from build123d import *

# Parameters (mm, degrees)
F1_DEPTH = 4.826
F3_DEPTH = 2.921
F5_DEPTH = 2.921
F7_DEPTH = 25.4
F8_R     = 3.302
F9_R     = 6.35


with BuildPart() as f1:
    # F0 (on Top) → F1 (new body)
    with BuildSketch(Plane.XY):
        Polygon((-9.795272, 20.32), (-15.24, 0), (15.24, 0), (9.795272, 20.32), align=None)
    extrude(amount=F1_DEPTH)

    # F2 (on face) → F3 (join)
    with BuildSketch(Plane.XY.offset(4.826)):
        Polygon((-19.841803, 0), (19.841803, 0), (12.185154, 28.575), (-12.185154, 28.575), align=None)
    extrude(amount=F3_DEPTH)

    # F4 (on face) → F5 (join)
    with BuildSketch(Plane(origin=(0, 0, 0), x_dir=(1, 0, 0), z_dir=(0, 0, -1))):
        Polygon((18.658482, 0), (-18.658482, 0), (-11.954661, -25.019), (11.954661, -25.019), align=None)
    extrude(amount=F5_DEPTH)

    # F6 (on face) → F7 (cut)
    with BuildSketch(Plane(origin=(0, 0, -2.921), x_dir=(1, 0, 0), z_dir=(0, 0, -1))):
        with BuildLine():
            Line((3.81, -8.255), (-3.81, -8.255))
            ThreePointArc((-3.81, -8.255), (-8.255, -12.7), (-3.81, -17.145))
            Line((-3.81, -17.145), (3.81, -17.145))
            ThreePointArc((3.81, -17.145), (8.255, -12.7), (3.81, -8.255))
        make_face()
    extrude(amount=-F7_DEPTH, mode=Mode.SUBTRACT)

    # F8
    f8_edges = [f1.edges().sort_by_distance(p)[0] for p in [
        (9.795272, 20.32, 2.413),
        (-9.795272, 20.32, 2.413),
    ]]
    fillet(f8_edges, radius=F8_R)

    # F9
    f9_edges = [f1.edges().sort_by_distance(p)[0] for p in [
        (12.185154, 28.575, 6.2865),
        (-12.185154, 28.575, 6.2865),
        (11.954661, 25.019, -1.4605),
        (-11.954661, 25.019, -1.4605),
    ]]
    fillet(f9_edges, radius=F9_R)


solid = f1.part
Read the model definition and answer for the solid it produces. Units are mm, in the model's axes. A direction names the side the tool comes from. Round coordinates to 2 decimals unless told otherwise and drop trailing zeros. Order: outer loops, then holes, each group sorted by start corner. A loop starts at its lowest first (then second) coordinate and runs counter-clockwise, first axis right, second up. Notation, with made-up numbers: (32, -26.5) - (65, -26.5) arc R25 cw to (65, 11.5) - close; hole circle Ø7 at (62, -39). An arc over 180 degrees is marked (long way). Use one line per item in the form item = value. Start each with the question number.
(1) The part is cut by section A-A (z = 2.75). Give the vertices of the cut face in (x, y) (3 decimals), then the cut area to 3 significant figures.
(2) Determine the mould class of faces 4 (the face through (0, 18, 7.747)), 5 (the face through (-15.975, 10.014, -1.44)), 6 (the face through (8.254, 12.798, 2.338)) for opening direction X: +X half, -X half, draft (parallel to the pull), parting line (faces both ways), or undercut.
(3) For faces 1 (the face through (-12.8, 9.1, 2.4)), 2 (the face through (0, 21, 4.826)), 3 (the face through (9.296, 19.619, 2.447)), determine the directions among +Z, -Z, +X, -X, +Y, -Y from which every point of the face is accessible in a straight line to the end or side of a thin tool.
(4) Find the intervals of material crossed by line 1 along Z through (x, y) = (10, 19); line 2 along X through (y, z) = (16.5, 5.5); line 3 along X through (y, z) = (9.25, 7.25), in increasing order. Write a range as from..to.
(5) Flat-ended cylindrical pins translate along their axes: pin 1 Ø5 at (y, z) = (21, -1) entering from -X; pin 2 Ø5.5 at (x, z) = (2.5, 1.5) entering from +Y; pin 3 Ø2 at (x, z) = (-14, 0) entering from -Y; pin 4 Ø6 at (y, z) = (16.5, 5.5) entering from -X. Find the tip coordinate at first contact, or state that the pin passes through.
(6) The part is cut by section B-B (y = 10). Give the vertices of the cut face in (x, z).
(7) The part is cut by section D-D (x = 11). Give the vertices of the cut face in (y, z).
Checked values:
q1.outline = (-15.24, 0) - (15.24, 0) - (10.451, 17.873) arc R3.302 ccw to (7.262, 20.32) - (-7.262, 20.32) arc R3.302 ccw to (-10.451, 17.873) - close; hole (-3.81, 8.255) - (3.81, 8.255) arc R4.445 ccw to (3.81, 17.145) - (-3.81, 17.145) arc R4.445 ccw to start
q1.area = 376 mm^2
q2.face_4 = draft
q2.face_5 = -X half
q2.face_6 = undercut
q3.face_1 = -X, +Y
q3.face_2 = +Y
q3.face_3 = +X, +Y
q4.line_1 = -2.92..0, 4.83..7.75
q4.line_2 = -15.42..-6.12, 6.12..15.42
q4.line_3 = -17.36..-6.61, 6.61..17.36
q5.pin_1 = -13.7
q5.pin_2 = 25.02
q5.pin_3 = 0
q5.pin_4 = -16.22
q6.outline = (-17.16, 4.83) - (-12.56, 4.83) - (-12.56, 0) - (-15.98, 0) - (-15.98, -2.92) - (-7.34, -2.92) - (-7.34, 7.75) - (-17.16, 7.75) - close; (7.34, -2.92) - (15.98, -2.92) - (15.98, 0) - (12.56, 0) - (12.56, 4.83) - (17.16, 4.83) - (17.16, 7.75) - (7.34, 7.75) - close
q7.outline = (0, -2.92) - (23.67, -2.92) - (23.67, 0) - (15.82, 0) - (15.82, 4.83) - (27.39, 4.83) - (27.39, 7.75) - (0, 7.75) - close
